Answer from the drawing. Dimensions are ordinates in mm from the lowest x, y and z of the part. A direction names the side the tool comes from. Coordinates: 2 decimals unless noted, no trailing zeros. Write each loop counter-clockwise with the first axis right and the second up, starting at its lowest first coordinate (ties: lowest second). Pieces come first, ordered by that corner, then holes.
(1) The part is cut by section B-B on y = 2.3. Determine the outline of the cut face in (x, z).
(2) Which of the six approach directions +Z, -Z, +X, -X, +Y, -Y give full straight-line access (tool end or side, diameter ignored) to the marked faces 4 and 5?
(3) The part is cut by section C-C on z = 31.5. Determine the outline of the cut face in (x, y).
(4) The part is cut by section D-D on x = 5. Determine the outline of the cut face in (y, z), plus the area to 3 significant figures.
(5) Straight lines are drawn through the part: line 1 (Z direction, x = 17.5, y = 1.65); line 2 (X direction, y = 4, z = 18); line 3 (X direction, y = 0.3, z = 14). For each, find the intervals that lie inside material, in ascending order.
(6) The part is cut by section A-A on x = 18. Determine the outline of the cut face in (y, z), plus the area to 3 significant figures.
(7) Given P1, Ø1, axis at x = 28, y = 4, coming from the +Z side; P2, Ø2, axis at y = 3, z = 9, coming from the +X side, each flat-ended and moving along its own axis, determine where each tip first touches the part or whether it passes through.
(8) For a pull along X with two mould halves and no side action, classify the marked faces 1, 2 and 3 as +X half, -X half, draft (parallel to the pull), parting line (faces both ways), or undercut.
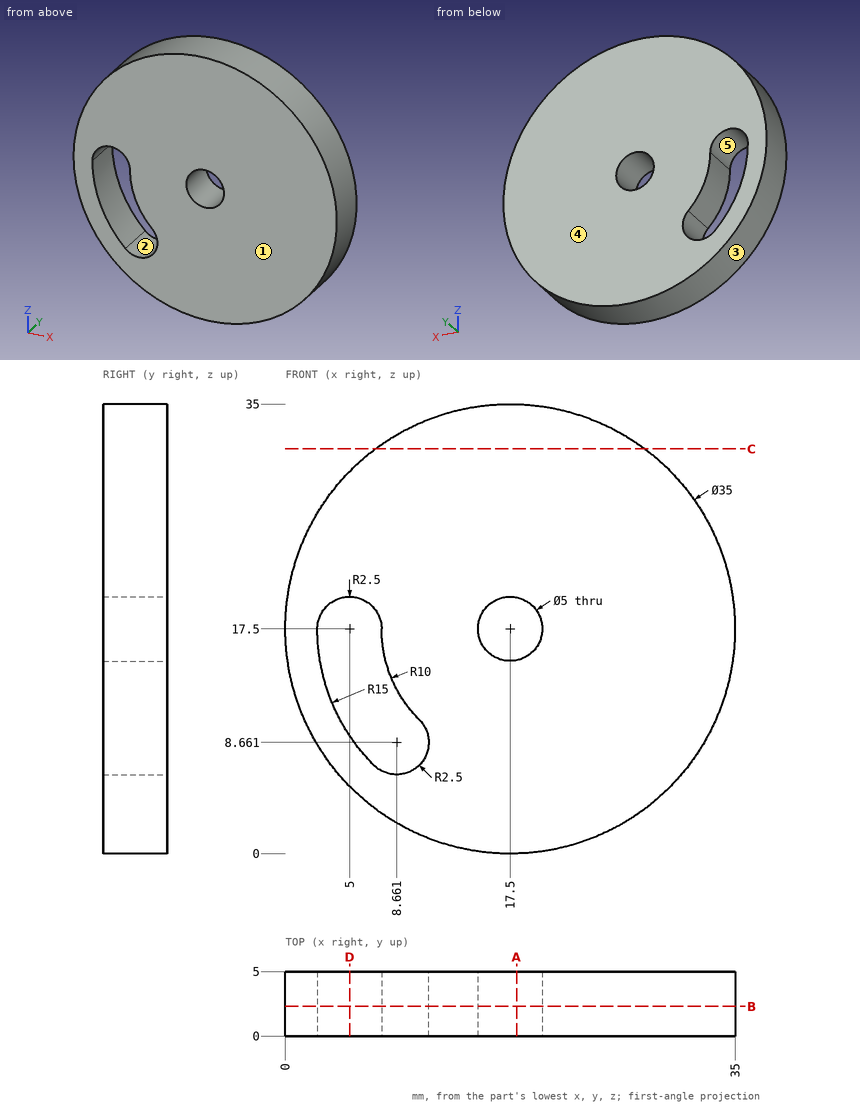
Model answer:
1. outline: circle Ø35 at (17.5, 17.5); hole (2.5, 17.5) arc R15 ccw to (6.89, 6.89) arc R2.5 ccw to (10.43, 10.43) arc R10 cw to (7.5, 17.5) arc R2.5 ccw to start; hole circle Ø5 at (17.5, 17.5)
2. face 4: +Z, -Z, +X, -X, +Y
2. face 5: +Y, -Y
3. outline: (7, 0) - (28, 0) - (28, 5) - (7, 5) - close
4. outline: (0, 5.25) - (5, 5.25) - (5, 9.21) - (0, 9.21) - close; (0, 20) - (5, 20) - (5, 29.75) - (0, 29.75) - close
4. area: 68.5 mm2
5. line 1: z = 0 to 15, 20 to 35
5. line 2: x = 0.01 to 2.55, 7.45 to 15.05, 19.95 to 34.99
5. line 3: x = 0.35 to 2.91, 8.13 to 34.65
6. outline: (0, 0.01) - (5, 0.01) - (5, 15.05) - (0, 15.05) - close; (0, 19.95) - (5, 19.95) - (5, 34.99) - (0, 34.99) - close
6. area: 150 mm2
7. P1: stops at z = 31.86
7. P2: stops at x = 33.31
8. face 1: draft
8. face 2: undercut
8. face 3: parting line
